The listing builds one solid part. Answer for the finished solid, in the listing's coordinates (mm). A direction names the side the tool comes from. Give positions to 0.01 mm unless a question says otherwise; leave off trailing zeros. Write each loop counter-clockwise with the first axis right and the second up, starting at its lowest first coordinate (ties: lowest second). Pieces come first, ordered by that corner, then holes.
```python
from build123d import *

# Parameters (mm, degrees)
F3_DEPTH = 40.001


with BuildPart() as f1:
    # F0 (on Right) → F1 (revolve)
    with BuildSketch(Plane.YZ):
        Polygon((-20, 25), (0, 25), (20, 25), (20, 275), (12.558388, 275), (10, 255.164309), (0, 255.164309), (-10, 255.164309), (-12.558388, 275), (-20, 275), align=None)
    revolve(axis=Axis((0, 0.25152, 0), (0, 1, 0)))

    # F2 (on face) → F3 (cut, through all)
    with BuildSketch(Plane.XZ.offset(20)):
        Polygon((0, 33.918292), (-6, 33.918292), (-6, 23.918292), (0, 23.918292), (6, 23.918292), (6, 33.918292), align=None)
    extrude(amount=-F3_DEPTH, mode=Mode.SUBTRACT)


solid = f1.part
```
Item 1: Determine the mould class of faces 1 (the face through (76.934, 10.124, 244.3)), 2 (the face through (-57, -20, -4)), 3 (the face through (-57, 20, 4)) for opening direction Y: pulls with the +Y half, pulls with the -Y half, needs draft (parallel to the pull), parting line crosses it, or undercut.
Conclusion:
face 1: undercut
face 2: pulls with the -Y half
face 3: pulls with the +Y half
Item 2: A cutting plane is placed at A-A, the plane y = 0. Give the vertices of the cut face in (x, z).
Conclusion:
outline: circle Ø510.33 at (0, 0); hole (-6, 24.27) arc R25 ccw (long way) to (6, 24.27) - (6, 33.92) - (-6, 33.92) - close
Item 3: Each of these flat-tipped pins is pushed along its axis until it touches: P1, Ø3, axis at x = -77, y = 14.5, coming from the +Z side; P2, Ø1, axis at x = -92, y = -15.5, coming from the +Z side; P3, Ø6, axis at x = -139, y = -2, coming from the +Z side. Where does it stop, or does it pass through?
Conclusion:
P1: stops at z = 264.43
P2: stops at z = 259.33
P3: stops at z = 215.9
Item 4: Which of the six approach directions +Z, -Z, +X, -X, +Y, -Y give full straight-line access (tool end or side, diameter ignored) to faces 4 (the face through (0, 0, 33.918)), 5 (the face through (77.02, -10.16, 244.56))?
Conclusion:
face 4: +Y, -Y
face 5: none
Item 5: Consider probe 1 along X at (y, z) = (5, 0); probe 2 along X at (y, z) = (17.5, -11); probe 3 along Z at (x, y) = (-114.5, -9). Determine where each line is inside the solid, lowest interval first.
Conclusion:
probe 1: x = -255.16 to -25, 25 to 255.16
probe 2: x = -274.78 to -22.45, 22.45 to 274.78
probe 3: z = -228.03 to 228.03
